Could you check a few things on this model? Use its own coordinates, in mm. Round coordinates to 2 decimals unless told otherwise and drop trailing zeros. Loops run counter-clockwise (first coordinate to the right, second up) from the corner with the lowest first, then second, coordinate; pieces in that order, holes last. Notation, with made-up numbers: (-25, 9.5) -> (25, 9.5) arc R19 ccw to (25, 19.5) -> close; hole circle Ø2 at (59.5, 76.5). An arc over 180 degrees is marked (long way). One line per item, written item: value.
from build123d import *

# Parameters (mm, degrees)
F0_W      = 9.525
F0_H      = 19.05
F0_R      = 2.15265
F1_DEPTH  = 15.875
F2_W      = 9.525
F2_H      = 3.175
F3_DEPTH  = 9.525
F4_R      = 2.15265
F5_DEPTH  = 9.525
F3_FACE_W = 9.525
F3_FACE_H = 3.175
F6_DEPTH  = 9.525


with BuildPart() as f1:
    # F0 (on Top) → F1 (new body)
    with BuildSketch(Plane.XY):
        with Locations((4.7625, 9.525)):
            Rectangle(F0_W, F0_H)
        with Locations((4.7625, 14.2875)):
            Circle(F0_R, mode=Mode.SUBTRACT)
    extrude(amount=F1_DEPTH)

    # F2 (on face) → F3 (cut)
    with BuildSketch(Plane(origin=(0, 19.05, 0), x_dir=(-1, 0, 0), z_dir=(0, 1, 0))):
        with Locations((-4.7625, 1.5875)):
            Rectangle(F2_W, F2_H)
        with Locations((-4.7625, 14.2875)):
            Rectangle(F2_W, F2_H)
    extrude(amount=-F3_DEPTH, mode=Mode.SUBTRACT)

    # F4 (on face) → F5 (cut, through all)
    with BuildSketch(Plane(origin=(0, 0, 0), x_dir=(0, -1, 0), z_dir=(-1, 0, 0))):
        with Locations((-4.7625, 7.9375)):
            Circle(F4_R)
    extrude(amount=-F5_DEPTH, mode=Mode.SUBTRACT)

    # F3_face (on face) → F6 (cut, through all)
    with BuildSketch(Plane(origin=(4.7625, 9.525, 14.2875), x_dir=(-1, 0, 0), z_dir=(0, 1, 0))):
        Rectangle(F3_FACE_W, F3_FACE_H)
    extrude(amount=-F6_DEPTH, mode=Mode.SUBTRACT)


solid = f1.part
(1) If I drill on L1, parallel to Y at x = 2, z = 8; L2, parallel to Y at x = 6.25, z = 7; L3, parallel to Y at x = 6, z = 11.25, over which ranges is the centre line in solid material (lowest first)?
Recorded:
L1: 0 to 2.61, 6.91 to 19.05
L2: 0 to 2.82, 6.7 to 12.73, 15.84 to 19.05
L3: 0 to 12.53, 16.05 to 19.05
(2) I'm going to push flat-ended pins straight in: pin 1 Ø2.5 at (y, z) = (4.76, 7.94) entering from -X; pin 2 Ø1 at (x, z) = (3, 2) entering from +Y (3 decimals). Where does each tip first touch, or does it pass through?
Recorded:
pin 1: through
pin 2: y = 9.525
(3) Thinking about a two-plate mould opening in Y: for faces 1 (the face through (5, 9.525, 2)), 2 (the face through (5.92, 16.103, 7.871)), 3 (the face through (7, 15, 3.175)), 4 (the face through (5, 0, 6)), which applies, released by +Y, released by -Y, zero draft, split by the parting line, or undercut?
Recorded:
face 1: released by +Y
face 2: undercut
face 3: zero draft
face 4: released by -Y
(4) If we section it at A-A, the plane x = 4.75: Give the number of separate pieces and of enclosed holes in the cut face, then the cut area to 3 significant figures.
Recorded:
separate pieces: 2
enclosed holes: 1
area: 156 mm²
(5) If we section it at C-C, the plane y = 16: Please give me the cut outline in (x, z) (3 decimals), then the cut area to 3 significant figures.
Recorded:
outline: (0, 3.175) -> (3.458, 3.175) -> (3.458, 12.7) -> (0, 12.7) -> close; (6.067, 3.175) -> (9.525, 3.175) -> (9.525, 12.7) -> (6.067, 12.7) -> close
area: 65.9 mm²
